from build123d import *

# Parameters (mm, degrees)
F0_W     = 152.4
F0_H     = 127
F1_DEPTH = 76.2
F2_W     = 127
F2_H     = 101.6
F3_DEPTH = 50.8
F4_R     = 5.08


with BuildPart() as f1:
    # F0 (on Front) → F1 (new body)
    with BuildSketch(Plane.XZ):
        Rectangle(F0_W, F0_H)
    extrude(amount=-F1_DEPTH)

    # F2 (on face) → F3 (cut)
    with BuildSketch(Plane.XZ):
        Rectangle(F2_W, F2_H)
    extrude(amount=-F3_DEPTH, mode=Mode.SUBTRACT)

    # F4
    f4_edges = [f1.edges().sort_by_distance(p)[0] for p in [
        (-76.2, 0, 0),
        (0, 0, 63.5),
        (0, 0, 50.8),
        (-63.5, 0, 0),
        (0, 0, -50.8),
        (0, 0, -63.5),
        (76.2, 0, 0),
        (63.5, 0, 0),
        (76.2, 38.1, 63.5),
        (76.2, 76.2, 0),
        (76.2, 38.1, -63.5),
        (-76.2, 38.1, 63.5),
        (0, 76.2, 63.5),
        (-76.2, 38.1, -63.5),
        (-76.2, 76.2, 0),
        (0, 76.2, -63.5),
    ]]
    fillet(f4_edges, radius=F4_R)


solid = f1.part
Geometry check sheet. Reference: the model listing, model coordinates, mm. A direction names the side the tool comes from. Coordinates: 2 decimals unless noted, no trailing zeros. Order: outer loops, then holes, each group sorted by start corner. A loop starts at its lowest first (then second) coordinate and runs counter-clockwise, first axis right, second up. Notation, with made-up numbers: (-15, 15.25) -> (8, 15.25) arc R19 ccw to (8, 49.25) -> close; hole circle Ø7 at (77.5, 38.5). An arc over 180 degrees is marked (long way). Use a Markdown table: item, result. Add a question column.
1. Cross-section at A-A (y = 37). Enter the section's corners in (x, z).
2. Material ranges on L1, parallel to Z at x = 41, y = 25.5; L2, parallel to X at y = 17, z = 36.5; L3, parallel to Y at x = 11, z = -34, recorded low to high.
3. Cross-section at C-C (z = 28.5). Enter the section's corners in (x, y), and give its area (3 significant figures).
4. Go/stop test with a flat-tipped pin: pin 1 Ø10 at (x, z) = (-17, -26) entering from -Y. Record where the tip stops, or that it passes through.
5. Cross-section at B-B (x = -15). Enter the section's corners in (y, z), and give its area (3 significant figures).
6. Set-up check for faces 1 (the face through (0.96, 1.449, -52.328)), 2 (the face through (74.672, 38.562, -62.051)): record each of +Z, -Z, +X, -X, +Y, -Y from which the full face is reachable in a straight line by a thin tool's end or side.
7. Mould release check, pull along X, two halves, no side actions. Record for faces 3 (the face through (0.996, 1.528, 62.051)), 4 (the face through (-1, 28, -50.8)), 5 (the face through (-74.751, 38.562, -61.972)): pulls with the +X half, pulls with the -X half, needs draft (parallel to the pull), parting line crosses it, or undercut.
Filled sheet:
| question | item | result |
|---|---|---|
| 1 | outline | (-76.2, -58.42) arc R5.08 ccw to (-71.12, -63.5) -> (71.12, -63.5) arc R5.08 ccw to (76.2, -58.42) -> (76.2, 58.42) arc R5.08 ccw to (71.12, 63.5) -> (-71.12, 63.5) arc R5.08 ccw to (-76.2, 58.42) -> close; hole (-63.5, -50.8) -> (63.5, -50.8) -> (63.5, 50.8) -> (-63.5, 50.8) -> close |
| 2 | L1 | -63.5 to -50.8, 50.8 to 63.5 |
| 2 | L2 | -76.2 to -63.5, 63.5 to 76.2 |
| 2 | L3 | 50.8 to 76.2 |
| 3 | outline | (-76.2, 5.08) arc R5.08 ccw to (-71.12, 0) -> (-68.58, 0) arc R5.08 ccw to (-63.5, 5.08) -> (-63.5, 50.8) -> (63.5, 50.8) -> (63.5, 5.08) arc R5.08 ccw to (68.58, 0) -> (71.12, 0) arc R5.08 ccw to (76.2, 5.08) -> (76.2, 71.12) arc R5.08 ccw to (71.12, 76.2) -> (-71.12, 76.2) arc R5.08 ccw to (-76.2, 71.12) -> close |
| 3 | area | 5,130 mm2 |
| 4 | pin 1 | y = 50.8 |
| 5 | outline | (0, -58.42) arc R5.08 ccw to (5.08, -63.5) -> (71.12, -63.5) arc R5.08 ccw to (76.2, -58.42) -> (76.2, 58.42) arc R5.08 ccw to (71.12, 63.5) -> (5.08, 63.5) arc R5.08 ccw to (0, 58.42) -> (0, 55.88) arc R5.08 ccw to (5.08, 50.8) -> (50.8, 50.8) -> (50.8, -50.8) -> (5.08, -50.8) arc R5.08 ccw to (0, -55.88) -> close |
| 5 | area | 4,480 mm2 |
| 6 | face 1 | -Y |
| 6 | face 2 | -Z, +X, +Y, -Y |
| 7 | face 3 | needs draft |
| 7 | face 4 | undercut |
| 7 | face 5 | pulls with the -X half |
